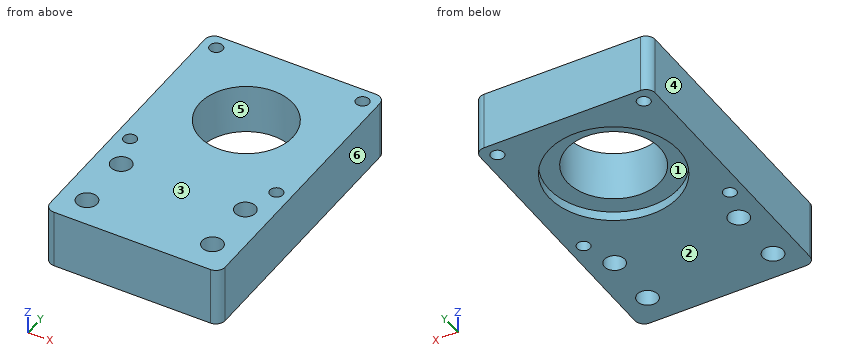
from build123d import *

# Parameters (mm, degrees)
SKETCH1_W               = 56.4
SKETCH1_H               = 56.4
BOSS_EXTRUDE1_DEPTH     = 19
SKETCH2_R               = 20.904355549
CUT_EXTRUDE2_DEPTH      = 20
SKETCH3_W               = 56.4
SKETCH3_H               = 34.3
BOSS_EXTRUDE2_DEPTH     = 19
FILLET1_R               = 3
TAP_DRILL_FOR_M5_TAP1_D = 4.2
M6_CLEARANCE_HOLE1_D    = 6.6
SKETCH8_R               = 20.904355549
SKETCH8_R_2             = 15
BOSS_EXTRUDE3_DEPTH     = 16


with BuildPart() as part:
    # Sketch1 → Boss-Extrude1 (new body)
    with BuildSketch(Plane.XY):
        with Locations((0, 25)):
            Rectangle(SKETCH1_W, SKETCH1_H)
    extrude(amount=BOSS_EXTRUDE1_DEPTH)

    # Sketch2 → Cut-Extrude2 (cut)
    with BuildSketch(Plane.XY.offset(19)):
        with Locations((0, 25)):
            Circle(SKETCH2_R)
    extrude(amount=-CUT_EXTRUDE2_DEPTH, mode=Mode.SUBTRACT)

    # Sketch3 → Boss-Extrude2 (add)
    with BuildSketch(Plane(origin=(0, 0, 0), x_dir=(-1, 0, 0), z_dir=(0, 0, -1))):
        with Locations((0, -20.35)):
            Rectangle(SKETCH3_W, SKETCH3_H)
    extrude(amount=-BOSS_EXTRUDE2_DEPTH)

    # Fillet1
    fillet1_edges = [part.edges().sort_by_distance(p)[0] for p in [
        (28.2, -37.5, 9.5),
        (-28.2, -37.5, 9.5),
        (28.2, 53.2, 9.5),
        (-28.2, 53.2, 9.5),
    ]]
    fillet(fillet1_edges, radius=FILLET1_R)

    # Tap Drill for M5 Tap1 (through all)
    with Locations(Plane(origin=(0, 0, 0), x_dir=(-1, 0, 0), z_dir=(0, 0, -1))):
        with Locations((-23.57, 48.57), (23.57, 48.57), (-23.57, 1.43), (23.57, 1.43)):
            Hole(TAP_DRILL_FOR_M5_TAP1_D / 2)

    # M6 Clearance Hole1 (through all)
    with Locations(Plane(origin=(0, 0, 0), x_dir=(-1, 0, 0), z_dir=(0, 0, -1))):
        with Locations((-20, -9.5), (-20, -27.5), (20, -28.237657735), (20, -9.5)):
            Hole(M6_CLEARANCE_HOLE1_D / 2)

    # Sketch8 → Boss-Extrude3 (add)
    with BuildSketch(Plane.XY.offset(19)):
        with Locations((0, 25)):
            Circle(SKETCH8_R)
        with Locations((0, 25)):
            Circle(SKETCH8_R_2, mode=Mode.SUBTRACT)
    extrude(amount=-BOSS_EXTRUDE3_DEPTH)


solid = part.part
Work out the finished part from the listing and answer in its coordinate system (mm). Face numbers are marked on the shaded views. A direction names the side the tool comes from. Coordinates: 2 decimals unless noted, no trailing zeros. Write each loop counter-clockwise with the first axis right and the second up, starting at its lowest first coordinate (ties: lowest second). Pieces come first, ordered by that corner, then holes.
1. For the marked faces 1 and 2, determine the directions among +Z, -Z, +X, -X, +Y, -Y from which every point of the face is accessible in a straight line to the end or side of a thin tool.
Results list:
face 1: -Z
face 2: -Z, +X, -X, +Y, -Y
2. The part is cut by section B-B, the plane x = 20. Write down the section's boundary in (y, z).
Results list:
outline: (-37.5, 0) - (-30.8, 0) - (-30.8, 19) - (-37.5, 19) - close; (-24.2, 0) - (-12.8, 0) - (-12.8, 19) - (-24.2, 19) - close; (-6.2, 0) - (18.92, 0) - (18.92, 3) - (31.08, 3) - (31.08, 0) - (53.2, 0) - (53.2, 19) - (-6.2, 19) - close
3. The part is cut by section D-D, the plane z = 17. State how many separate pieces and enclosed holes the cut face has, and give its area (3 significant figures).
Results list:
separate pieces: 1
enclosed holes: 9
area: 4,210 mm2
4. For a pull along X with two mould halves and no side action, classify the marked faces 3, 4, 5 and 6 as +X half, -X half, draft (parallel to the pull), parting line (faces both ways), or undercut.
Results list:
face 3: draft
face 4: -X half
face 5: undercut
face 6: +X half
5. The part is cut by section A-A, the plane y = 25. Write down the section's boundary in (x, z).
Results list:
outline: (-28.2, 0) - (-20.9, 0) - (-20.9, 3) - (-15, 3) - (-15, 19) - (-28.2, 19) - close; (15, 3) - (20.9, 3) - (20.9, 0) - (28.2, 0) - (28.2, 19) - (15, 19) - close
6. Consider line 1 along Y through (x, z) = (-20, 7.25); line 2 along Y through (x, z) = (20, 11.5); line 3 along X through (y, z) = (-26.5, 14.25). Determine where each line is inside the solid, lowest interval first.
Results list:
line 1: y = -37.5 to -31.54, -24.94 to -12.8, -6.2 to 53.2
line 2: y = -37.5 to -30.8, -24.2 to -12.8, -6.2 to 53.2
line 3: x = -28.2 to -22.81, -17.19 to 16.86, 23.14 to 28.2
7. The part is cut by section C-C, the plane y = -9.5. Write down the section's boundary in (x, z), and give its area (3 significant figures).
Results list:
outline: (-28.2, 0) - (-23.3, 0) - (-23.3, 19) - (-28.2, 19) - close; (-16.7, 0) - (16.7, 0) - (16.7, 19) - (-16.7, 19) - close; (23.3, 0) - (28.2, 0) - (28.2, 19) - (23.3, 19) - close
area: 821 mm2
8. Flat-ended cylindrical pins translate along their axes: pin 1 (5.5 mm diameter, centred on x = -20, y = -28.24, fed in from +Z); pin 2 (21 mm diameter, centred on x = 6, y = 23.5, fed in from -Z). Find the tip coordinate at first contact, or state that the pin passes through.
Results list:
pin 1: passes through
pin 2: stops at z = 3
